```python
from build123d import *

# Parameters (mm, degrees)
PAD_DEPTH          = 13.5
SKETCH001_W        = 37.5
SKETCH001_H        = 61
POCKET_DEPTH       = 12
SKETCH002_W        = 13
SKETCH002_H        = 13.5
POCKET012020_DEPTH = 9.5
SKETCH004_W        = 12
SKETCH004_H        = 13.5
SKETCH004_W_2      = 12.5
POCKET012021_DEPTH = 4.5
SKETCH003_R        = 1.6
SKETCH003_R_2      = 1.2
POCKET012022_DEPTH = 9.001
SKETCH006_R        = 2.5
POCKET012023_DEPTH = 3
SKETCH007_R        = 1
POCKET012024_DEPTH = 1.5
POCKET012025_DEPTH = 40.501
PAD016_DEPTH       = 13
SKETCH019_W        = 9
SKETCH019_H        = 2
SKETCH019_W_2      = 4
POCKET012026_DEPTH = 1.501
POCKET012027_DEPTH = 9
POCKET012028_DEPTH = 4
CHAMFER_SIZE       = 0.8
FILLET001_R        = 0.8


with BuildPart() as part:
    # Sketch → Pad (new body)
    with BuildSketch(Plane.XY):
        Polygon((-19.25, 38.75), (19.25, 38.75), (20.25, 37.75), (20.25, -37.75), (19.25, -38.75), (-19.25, -38.75), (-20.25, -37.75), (-20.25, 37.75), align=None)
    extrude(amount=PAD_DEPTH)

    # Sketch001 → Pocket (cut)
    with BuildSketch(Plane.XY.offset(13.5)):
        with Locations((0, -6.75)):
            Rectangle(SKETCH001_W, SKETCH001_H)
    extrude(amount=-POCKET_DEPTH, mode=Mode.SUBTRACT)

    # Sketch002 → Pocket012020 (cut)
    with BuildSketch(Plane.XY.offset(13.5)):
        with Locations((0.25, 30.5)):
            Rectangle(SKETCH002_W, SKETCH002_H)
    extrude(amount=-POCKET012020_DEPTH, mode=Mode.SUBTRACT)

    # Sketch004 → Pocket012021 (cut)
    with BuildSketch(Plane.XY.offset(13.5)):
        with Locations((12.75, 30.5)):
            Rectangle(SKETCH004_W, SKETCH004_H)
        with Locations((-12.5, 30.5)):
            Rectangle(SKETCH004_W_2, SKETCH004_H)
    extrude(amount=-POCKET012021_DEPTH, mode=Mode.SUBTRACT)

    # Sketch003 → Pocket012022 (cut, through all)
    with BuildSketch(Plane.XY.offset(9)):
        with Locations((16.75, 29.25)):
            Circle(SKETCH003_R)
        with Locations((-9.75, 29.25)):
            Circle(SKETCH003_R)
        with Locations((9.75, 29.45)):
            Circle(SKETCH003_R_2)
    extrude(amount=-POCKET012022_DEPTH, mode=Mode.SUBTRACT)

    # Sketch006 → Pocket012023 (cut)
    with BuildSketch(Plane(origin=(0, 0, 0), x_dir=(1, 0, 0), z_dir=(0, 0, -1))):
        with Locations((16.75, -29.25)):
            Circle(SKETCH006_R)
        with Locations((-9.75, -29.25)):
            Circle(SKETCH006_R)
    extrude(amount=-POCKET012023_DEPTH, mode=Mode.SUBTRACT)

    # Sketch007 → Pocket012024 (cut)
    with BuildSketch(Plane.YZ.offset(20.25)):
        with Locations((24.9, 11.5)):
            Circle(SKETCH007_R)
        with Locations((-5, 11.5)):
            Circle(SKETCH007_R)
        with Locations((-8, 11.5)):
            Circle(SKETCH007_R)
        with BuildLine():
            Line((17.9, 13.5), (17.9, 9.5))
            Line((17.9, 9.5), (8.9, 9.5))
            Line((8.9, 11.3), (8.9, 9.5))
            Line((8.9, 11.3), (8.7, 11.3))
            ThreePointArc((6.7, 11.3), (7.7, 10.3), (8.7, 11.3))
            Line((6.5, 11.3), (6.7, 11.3))
            Line((6.5, 11.3), (6.5, 9.5))
            Line((-2.5, 9.5), (6.5, 9.5))
            Line((-2.5, 9.5), (-2.5, 13.5))
            Line((17.9, 13.5), (-2.5, 13.5))
        make_face()
    extrude(amount=-POCKET012024_DEPTH, mode=Mode.SUBTRACT)

    # Sketch017 → Pocket012025 (cut, through all)
    with BuildSketch(Plane.YZ.offset(20.25)):
        Polygon((38.773503, 10), (33, 0), (38.773503, 0), align=None)
    extrude(amount=-POCKET012025_DEPTH, mode=Mode.SUBTRACT)

    # Sketch018 → Pad016 (new body)
    with BuildSketch(Plane.YZ.offset(-6.25)):
        Polygon((37.25, 9), (37.25, 7.361216), (35.309401, 4), (34.363249, 4), align=None)
    extrude(amount=PAD016_DEPTH)

    # Sketch019 → Pocket012026 (cut, through all)
    with BuildSketch(Plane(origin=(0, -37.25, 0), x_dir=(-1, 0, 0), z_dir=(0, 1, 0))):
        with Locations((-12.75, 11)):
            Rectangle(SKETCH019_W, SKETCH019_H)
        with Locations((15.25, 11)):
            Rectangle(SKETCH019_W_2, SKETCH019_H)
    extrude(amount=-POCKET012026_DEPTH, mode=Mode.SUBTRACT)

    # Sketch022 → Pocket012027 (cut)
    with BuildSketch(Plane(origin=(17.25, 0, 0), x_dir=(0, -1, 0), z_dir=(-1, 0, 0))):
        Polygon((38.75, 12), (37.25, 13.5), (37.25, 12), align=None)
    extrude(amount=POCKET012027_DEPTH, mode=Mode.SUBTRACT)

    # Sketch039 → Pocket012028 (cut)
    with BuildSketch(Plane(origin=(-13.25, 0, 0), x_dir=(0, -1, 0), z_dir=(-1, 0, 0))):
        Polygon((38.75, 12), (37.25, 12), (37.25, 13.5), align=None)
    extrude(amount=POCKET012028_DEPTH, mode=Mode.SUBTRACT)

    # Chamfer
    chamfer_edges = [part.edges().sort_by_distance(p)[0] for p in [
        (0, -38.75, 0),
        (-19.75, -38.25, 0),
        (-20.25, -2.375, 0),
        (0, 33, 0),
        (20.25, -2.375, 0),
        (19.75, -38.25, 0),
    ]]
    chamfer(chamfer_edges, length=CHAMFER_SIZE)

    # Fillet001
    fillet001_edges = [part.edges().sort_by_distance(p)[0] for p in [
        (14.25, 29.25, 3),
        (-12.25, 29.25, 3),
    ]]
    fillet(fillet001_edges, radius=FILLET001_R)


solid = part.part
```
Design review of the part built by this model. Coordinates are the model's own, in mm. A direction names the side the tool comes from. Round coordinates to 2 decimals unless told otherwise and drop trailing zeros. Order: outer loops, then holes, each group sorted by start corner. A loop starts at its lowest first (then second) coordinate and runs counter-clockwise, first axis right, second up. Notation, with made-up numbers: (73, -34.75) - (95, -34.75) arc R15 cw to (95, -7.75) - close; hole circle Ø8 at (-23.75, -33.5). An arc over 180 degrees is marked (long way). Return JSON: item names as keys, results as strings.
Q1. The part is to be moulded in two halves that separate along Z. For faces 5 (the flat face through (0, -2, 0)), 6 (the flat face through (20, 6.5, 10)), 7 (the flat face through (-17.25, -38, 11)), say which applies: pulls with the +Z half, pulls with the -Z half, needs draft (parallel to the pull), parting line crosses it, or undercut.
Computed values:
{"face 5": "pulls with the -Z half", "face 6": "needs draft", "face 7": "undercut"}
Q2. Consider section B-B on y = -8. Write out the cut boundary in (x, z).
Computed values:
{"outline": "(-20.25, 0.8) - (-19.45, 0) - (19.45, 0) - (20.25, 0.8) - (20.25, 10.5) - (18.75, 10.5) - (18.75, 1.5) - (-18.75, 1.5) - (-18.75, 13.5) - (-20.25, 13.5) - close; (18.75, 12.5) - (20.25, 12.5) - (20.25, 13.5) - (18.75, 13.5) - close"}
Q3. Consider section A-A on x = 9.75. Write out the cut boundary in (y, z).
Computed values:
{"outline": "(-38.75, 0.8) - (-37.95, 0) - (28.25, 0) - (28.25, 9) - (23.75, 9) - (23.75, 1.5) - (-37.25, 1.5) - (-37.25, 10) - (-38.75, 10) - close; (-38.75, 12) - (-37.25, 13.5) - (-38.75, 13.5) - close; (30.65, 0) - (32.2, 0) - (33.4, 0.69) - (38.75, 9.96) - (38.75, 13.5) - (37.25, 13.5) - (37.25, 9) - (30.65, 9) - close"}
Q4. Wall thickness on L1, parallel to X at y = 11, z = 6.5; L2, parallel to Z at x = 19.45, y = 24.9; L3, parallel to Y at x = 9, z = 4.5: over which ranges is each line inside the solid? List them lowest first. Write a range as [from, to].
Computed values:
{"L1": "x = [-20.25, -18.75], [18.75, 20.25]", "L2": "z = [0, 10.5], [12.5, 13.5]", "L3": "y = [-38.75, -37.25], [23.75, 28.51], [30.39, 35.6]"}
Q5. Machinability: for faces 1 (the flat face through (-18.75, -9, 8)), 2 (the flat face through (8.25, -38, 11)), 3 (the flat face through (20, 17.9, 12)), 4 (the cylindrical face through (-10.08, 26.77, 1.08)), which of the approach directions +Z, -Z, +X, -X, +Y, -Y give a long, thin tool a straight path to every point of the face, cutting with its end or side? Answer none if there is none.
Computed values:
{"face 1": "+Z", "face 2": "none", "face 3": "+Z, +X", "face 4": "-Z"}
Q6. For pin 1 Ø4.5 at (x, y) = (16.75, 29.25) entering from +Z; pin 2 Ø6 at (x, y) = (12, 29.5) entering from +Z; pin 3 Ø5 at (x, y) = (-13.5, 2) entering from +Z; pin 4 Ø2.5 at (x, y) = (-10, 30) entering from -Z, all flat-tipped, find the tip position at first contact; note any pin that passes through.
Computed values:
{"pin 1": "stops at z = 13.5", "pin 2": "stops at z = 9", "pin 3": "stops at z = 1.5", "pin 4": "stops at z = 2.92"}
Q7. Consider section C-C on x = -9.75. Write out the cut boundary in (y, z).
Computed values:
{"outline": "(-38.75, 0.8) - (-37.95, 0) - (26.75, 0) - (26.75, 2.2) arc R0.8 cw to (27.55, 3) - (27.65, 3) - (27.65, 9) - (23.75, 9) - (23.75, 1.5) - (-37.25, 1.5) - (-37.25, 13.5) - (-38.75, 13.5) - close; (30.85, 3) - (30.95, 3) arc R0.8 cw to (31.75, 2.2) - (31.75, 0) - (32.2, 0) - (33.4, 0.69) - (38.75, 9.96) - (38.75, 13.5) - (37.25, 13.5) - (37.25, 9) - (30.85, 9) - close"}
Q8. Consider section D-D on z = 5.75. Write out the cut boundary in (x, y).
Computed values:
{"outline": "(-20.25, -37.75) - (-19.25, -38.75) - (19.25, -38.75) - (20.25, -37.75) - (20.25, 36.32) - (-20.25, 36.32) - close; hole (-18.75, -37.25) - (18.75, -37.25) - (18.75, 23.75) - (6.75, 23.75) - (6.75, 35.37) - (-6.25, 35.37) - (-6.25, 23.75) - (-18.75, 23.75) - close; hole circle Ø3.2 at (-9.75, 29.25); hole circle Ø2.4 at (9.75, 29.45); hole circle Ø3.2 at (16.75, 29.25)"}
